The listing builds one solid part. Answer for the finished solid, in the listing's coordinates (mm). A direction names the side the tool comes from. Round coordinates to 2 decimals unless told otherwise and drop trailing zeros. Loops run counter-clockwise (first coordinate to the right, second up) from the corner with the lowest first, then second, coordinate; pieces in that order, holes last. Notation, with made-up numbers: (-19.5, 23.25) - (21.5, 23.25) arc R15 cw to (21.5, 47.25) - close; hole circle Ø4 at (23, 46.25). An arc over 180 degrees is marked (long way). One line per item, written item: value.
```python
from build123d import *

# Parameters (mm, degrees)
F1_DEPTH = 6
F2_R     = 0.75
F3_DEPTH = 25
F4_W     = 1.5
F4_H     = 4.4
F5_DEPTH = 25


with BuildPart() as f1:
    # F0 (on Front) → F1 (new body)
    with BuildSketch(Plane.XZ):
        with BuildLine():
            Line((0, 2), (0, 0))
            Line((0, 0), (20, 0))
            Line((20, 0), (20, 2))
            ThreePointArc((20, 2), (10, 1.160798), (0, 2))
        make_face()
    extrude(amount=-F1_DEPTH)

    # F2 (on face) → F3 (cut)
    with BuildSketch(Plane(origin=(0, 0, 0), x_dir=(1, 0, 0), z_dir=(0, 0, -1))):
        with Locations((10, -3)):
            Circle(F2_R)
    extrude(amount=-F3_DEPTH, mode=Mode.SUBTRACT)

    # F4 (on face) → F5 (cut)
    with BuildSketch(Plane(origin=(0, 0, 0), x_dir=(1, 0, 0), z_dir=(0, 0, -1))):
        with Locations((5.45, -3)):
            Rectangle(F4_W, F4_H)
        with Locations((2.35, -3)):
            Rectangle(F4_W, F4_H)
        with Locations((14.55, -3)):
            Rectangle(F4_W, F4_H)
        with Locations((17.65, -3)):
            Rectangle(F4_W, F4_H)
    extrude(amount=-F5_DEPTH, mode=Mode.SUBTRACT)


solid = f1.part
```
1) A cutting plane is placed at B-B on y = 3. Give the vertices of the cut face in (x, z).
Final values:
outline: (0, 0) - (1.6, 0) - (1.6, 1.75) arc R60 cw to (0, 2) - close; (3.1, 0) - (4.7, 0) - (4.7, 1.4) arc R60 cw to (3.1, 1.56) - close; (6.2, 0) - (9.25, 0) - (9.25, 1.17) arc R60 cw to (6.2, 1.28) - close; (10.75, 0) - (13.8, 0) - (13.8, 1.28) arc R60 cw to (10.75, 1.17) - close; (15.3, 0) - (16.9, 0) - (16.9, 1.56) arc R60 cw to (15.3, 1.4) - close; (18.4, 0) - (20, 0) - (20, 2) arc R60 cw to (18.4, 1.75) - close
2) Consider L1, parallel to X at y = 3, z = 0.3; L2, parallel to X at y = 4.75, z = 0.4; L3, parallel to Y at x = 17, z = 0.1. Determine where each line is inside the solid, lowest interval first.
Final values:
L1: 0 to 1.6, 3.1 to 4.7, 6.2 to 9.25, 10.75 to 13.8, 15.3 to 16.9, 18.4 to 20
L2: 0 to 1.6, 3.1 to 4.7, 6.2 to 13.8, 15.3 to 16.9, 18.4 to 20
L3: 0 to 0.8, 5.2 to 6
3) A cutting plane is placed at C-C on z = 0.3. Give the vertices of the cut face in (x, y), and give its area (3 significant figures).
Final values:
outline: (0, 0) - (20, 0) - (20, 6) - (0, 6) - close; hole (1.6, 0.8) - (3.1, 0.8) - (3.1, 5.2) - (1.6, 5.2) - close; hole (4.7, 0.8) - (6.2, 0.8) - (6.2, 5.2) - (4.7, 5.2) - close; hole circle Ø1.5 at (10, 3); hole (13.8, 0.8) - (15.3, 0.8) - (15.3, 5.2) - (13.8, 5.2) - close; hole (16.9, 0.8) - (18.4, 0.8) - (18.4, 5.2) - (16.9, 5.2) - close
area: 91.8 mm2
4) This flat-tipped pin is pushed along its axis until it touches: pin 1 Ø1.5 at (x, y) = (5.5, 2.5) entering from +Z. Where does it stop, or does it pass through?
Final values:
pin 1: z = 1.28
5) For a pull along Y with two mould halves and no side action, classify faces 1 (the flat face through (10, 6, 1)), 2 (the flat face through (3.1, 3, 1)), 3 (the flat face through (0, 3, 1)), 4 (the flat face through (2, 5.2, 1)) as released by +Y, released by -Y, zero draft, split by the parting line, or undercut.
Final values:
face 1: released by +Y
face 2: undercut
face 3: zero draft
face 4: undercut
6) For faces 5 (the flat face through (13.8, 3, 1)), 6 (the cylindrical face through (10.14, 1.62, 1.16)), determine the directions among +Z, -Z, +X, -X, +Y, -Y from which every point of the face is accessible in a straight line to the end or side of a thin tool.
Final values:
face 5: +Z, -Z
face 6: +Z, +Y, -Y
7) A cutting plane is placed at D-D on y = 4.25. Give the vertices of the cut face in (x, z), and give its area (3 significant figures).
Final values:
outline: (0, 0) - (1.6, 0) - (1.6, 1.75) arc R60 cw to (0, 2) - close; (3.1, 0) - (4.7, 0) - (4.7, 1.4) arc R60 cw to (3.1, 1.56) - close; (6.2, 0) - (13.8, 0) - (13.8, 1.28) arc R60 cw to (6.2, 1.28) - close; (15.3, 0) - (16.9, 0) - (16.9, 1.56) arc R60 cw to (15.3, 1.4) - close; (18.4, 0) - (20, 0) - (20, 2) arc R60 cw to (18.4, 1.75) - close
area: 19.8 mm2
8) A cutting plane is placed at A-A on x = 10. Give the vertices of the cut face in (y, z).
Final values:
outline: (0, 0) - (2.25, 0) - (2.25, 1.16) - (0, 1.16) - close; (3.75, 0) - (6, 0) - (6, 1.16) - (3.75, 1.16) - close
